```python
from build123d import *

# Parameters (mm, degrees)
SKETCH1_W           = 25
SKETCH1_H           = 10
BOSS_EXTRUDE1_DEPTH = 10
SKETCH2_W           = 23
SKETCH2_H           = 7
CUT_EXTRUDE1_DEPTH  = 8
SKETCH3_R           = 1.5
CUT_EXTRUDE2_DEPTH  = 51
SKETCH4_R           = 2
CUT_EXTRUDE3_DEPTH  = 1
SKETCH5_R           = 1
CUT_EXTRUDE4_DEPTH  = 4


with BuildPart() as part:
    # Sketch1 → Boss-Extrude1 (new body)
    with BuildSketch(Plane.XY):
        Rectangle(SKETCH1_W, SKETCH1_H)
    extrude(amount=BOSS_EXTRUDE1_DEPTH)

    # Sketch2 → Cut-Extrude1 (cut)
    with BuildSketch(Plane(origin=(0, 0, 0), x_dir=(-1, 0, 0), z_dir=(0, 0, -1))):
        Rectangle(SKETCH2_W, SKETCH2_H)
    extrude(amount=-CUT_EXTRUDE1_DEPTH, mode=Mode.SUBTRACT)

    # Sketch3 → Cut-Extrude2 (cut)
    with BuildSketch(Plane(origin=(12.5, 0, 0), x_dir=(0, 0, -1), z_dir=(1, 0, 0))):
        with Locations((-5.152207195, 0)):
            Circle(SKETCH3_R)
    extrude(amount=-CUT_EXTRUDE2_DEPTH, mode=Mode.SUBTRACT)

    # Sketch4 → Cut-Extrude3 (cut)
    with BuildSketch(Plane(origin=(0, 0, 8), x_dir=(-1, 0, 0), z_dir=(0, 0, -1))):
        Circle(SKETCH4_R)
    extrude(amount=-CUT_EXTRUDE3_DEPTH, mode=Mode.SUBTRACT)

    # Sketch5 → Cut-Extrude4 (cut)
    with BuildSketch(Plane(origin=(0, 0, 9), x_dir=(-1, 0, 0), z_dir=(0, 0, -1))):
        Circle(SKETCH5_R)
    extrude(amount=-CUT_EXTRUDE4_DEPTH, mode=Mode.SUBTRACT)


solid = part.part
```
Read the model definition and answer for the solid it produces. Units are mm, in the model's axes. A direction names the side the tool comes from. Round coordinates to 2 decimals unless told otherwise and drop trailing zeros. Write each loop counter-clockwise with the first axis right and the second up, starting at its lowest first coordinate (ties: lowest second). Pieces come first, ordered by that corner, then holes. Notation, with made-up numbers: (46, 81.5) - (94, 81.5) arc R18 ccw to (94, 85.5) - close; hole circle Ø7 at (27, 25). An arc over 180 degrees is marked (long way). One line per item, written item: value.
Q1. For a pull along Z with two mould halves and no side action, classify faces 1 (the flat face through (0, 5, 5)), 2 (the cylindrical face through (-11.99, 0.45, 3.72)), 3 (the flat face through (-0.2, 1.2, 10)), 4 (the flat face through (0, 4, 0)) as pulls with the +Z half, pulls with the -Z half, needs draft (parallel to the pull), parting line crosses it, or undercut.
The answers:
face 1: needs draft
face 2: undercut
face 3: pulls with the +Z half
face 4: pulls with the -Z half
Q2. Find section B-B (z = 1). Determine the outline of the cut face in (x, y), and give its area (3 significant figures).
The answers:
outline: (-12.5, -5) - (12.5, -5) - (12.5, 5) - (-12.5, 5) - close; hole (-11.5, -3.5) - (11.5, -3.5) - (11.5, 3.5) - (-11.5, 3.5) - close
area: 89.0 mm2
Q3. Which of the six approach directions +Z, -Z, +X, -X, +Y, -Y give full straight-line access (tool end or side, diameter ignored) to faces 5 (the flat face through (0, 3.5, 4)), 6 (the cylindrical face through (0.217, -0.976, 9.493))?
The answers:
face 5: -Z
face 6: +Z, -Z
Q4. Straight lines are drawn through the part: line 1 (Y direction, x = 0, z = 9.8); line 2 (X direction, y = 2.25, z = 6); line 3 (Y direction, x = -10, z = 6.25). For each, find the intervals that lie inside material, in ascending order. Write a range as from..to.
The answers:
line 1: y = -5..-1, 1..5
line 2: x = -12.5..-11.5, 11.5..12.5
line 3: y = -5..-3.5, 3.5..5
Q5. Each of these flat-tipped pins is pushed along its axis until it touches: P1, Ø1.2, axis at x = -0.5, y = 0.5, coming from the -Z side; P2, Ø2.5, axis at y = 0, z = 5.15, coming from the +X side. Where does it stop, or does it pass through?
The answers:
P1: stops at z = 9
P2: passes through
Q6. Find section A-A (y = 0). Determine the outline of the cut face in (x, z), and give its area (3 significant figures).
The answers:
outline: (-12.5, 0) - (-11.5, 0) - (-11.5, 3.65) - (-12.5, 3.65) - close; (-12.5, 6.65) - (-11.5, 6.65) - (-11.5, 8) - (-2, 8) - (-2, 9) - (-1, 9) - (-1, 10) - (-12.5, 10) - close; (1, 9) - (2, 9) - (2, 8) - (11.5, 8) - (11.5, 6.65) - (12.5, 6.65) - (12.5, 10) - (1, 10) - close; (11.5, 0) - (12.5, 0) - (12.5, 3.65) - (11.5, 3.65) - close
area: 54.0 mm2
Q7. Find section D-D (y = 1.25). Determine the outline of the cut face in (x, z), and give its area (3 significant figures).
The answers:
outline: (-12.5, 0) - (-11.5, 0) - (-11.5, 4.32) - (-12.5, 4.32) - close; (-12.5, 5.98) - (-11.5, 5.98) - (-11.5, 8) - (-1.56, 8) - (-1.56, 9) - (1.56, 9) - (1.56, 8) - (11.5, 8) - (11.5, 5.98) - (12.5, 5.98) - (12.5, 10) - (-12.5, 10) - close; (11.5, 0) - (12.5, 0) - (12.5, 4.32) - (11.5, 4.32) - close
area: 59.6 mm2
Q8. Find section C-C (x = 0). Determine the outline of the cut face in (y, z).
The answers:
outline: (-5, 0) - (-3.5, 0) - (-3.5, 8) - (-2, 8) - (-2, 9) - (-1, 9) - (-1, 10) - (-5, 10) - close; (1, 9) - (2, 9) - (2, 8) - (3.5, 8) - (3.5, 0) - (5, 0) - (5, 10) - (1, 10) - close
